Here's how the part is built. I have some questions about the finished solid (model axes, mm). A direction names the side the tool comes from. Give positions to 0.01 mm unless a question says otherwise; leave off trailing zeros. Loops run counter-clockwise (first coordinate to the right, second up) from the corner with the lowest first, then second, coordinate; pieces in that order, holes last. Notation, with made-up numbers: (-18, 30.5) - (29, 30.5) arc R14 ccw to (29, 36.5) - close; hole circle Ø8 at (75, 41). An arc over 180 degrees is marked (long way). Put each result on its own line as item: value. Start each with the question number.
from build123d import *


# Not quite as in the source:
# - a fillet or chamfer that OpenCascade refuses, or shapes differently, is made with other operations: its cross-section is extruded or revolved along the edge and cut away or added


with BuildPart() as f1:
    # F0 (on Front) → F1 (revolve)
    with BuildSketch(Plane.XZ):
        Polygon((-30, 7), (-30, 0), (0, 0), (0, 50), (-11.6, 50), (-11.6, 52.4), (-16, 52.4), (-16, 50), (-14.085106383, 48.085106383), (-16, 5), (-25, 5), (-25, 7), align=None)
    revolve(axis=Axis((0, 0, 15.8572417056), (0, 0, 1)))

    # F2: fillet of radius 3 on 5 edges, made by hand

    # F2_s1 → F2_t2 (revolve)
    with BuildSketch(Plane.XZ):
        with BuildLine():
            ThreePointArc((-22.1715728753, 5), (-23.9036236828, 5.5505102572), (-25, 7))
            Line((-25, 7), (-25, 5))
            Line((-25, 5), (-22.1715728753, 5))
        make_face()
    revolve(axis=Axis((0, 0, 5), (0, 0, 1)))

    # F2_s3 → F2_t4 (revolve)
    with BuildSketch(Plane.XZ):
        with BuildLine():
            ThreePointArc((-14.1437787706, 46.764977662), (-14.3443716648, 47.9844003118), (-15.0194998464, 49.0194998464))
            Line((-15.0194998464, 49.0194998464), (-14.085106383, 48.085106383))
            Line((-14.085106383, 48.085106383), (-14.1437787706, 46.764977662))
        make_face()
    revolve(axis=Axis((0, 0, 48.085106383), (0, 0, 1)))

    # F2_s5 → F2_t6 (revolve)
    with BuildSketch(Plane.XZ):
        with BuildLine():
            ThreePointArc((-8.6606123087, 50), (-10.5579789048, 50.6762099923), (-11.6, 52.4))
            Line((-11.6, 52.4), (-11.6, 50))
            Line((-11.6, 50), (-8.6606123087, 50))
        make_face()
    revolve(axis=Axis((0, 0, 50), (0, 0, 1)))

    # F2_s7 → F2_t8 (revolve, cut)
    with BuildSketch(Plane.XZ):
        with BuildLine():
            ThreePointArc((-27, 7), (-29.1213203436, 6.1213203436), (-30, 4))
            Line((-30, 4), (-30, 7))
            Line((-30, 7), (-27, 7))
        make_face()
    revolve(axis=Axis((0, 0, 7), (0, 0, 1)), mode=Mode.SUBTRACT)

    # F2_s9 → F2_t10 (revolve, cut)
    with BuildSketch(Plane.XZ):
        with BuildLine():
            ThreePointArc((-16, 50), (-14.9579789048, 51.7237900077), (-13.0606123087, 52.4))
            Line((-13.0606123087, 52.4), (-16, 52.4))
            Line((-16, 52.4), (-16, 50))
        make_face()
    revolve(axis=Axis((0, 0, 52.4), (0, 0, 1)), mode=Mode.SUBTRACT)


solid = f1.part
1) I'm going to push flat-ended pins straight in: P1, Ø12, axis at x = 0, y = -21.5, coming from the +Z side; P2, Ø6, axis at x = 1.5, z = 21, coming from the +Y side; P3, Ø8, axis at x = 5, z = 38.5, coming from the -Y side. Where does each tip first touch, or does it pass through?
2) Thinking about a two-plate mould opening in Y: for faces 1 (the flat face through (0, 0, 50)), 2 (the flat face through (0, -12, 52.4)), 3 (the cylindrical face through (29.97, -1.32, 1.97)), which applies, pulls with the +Y half, pulls with the -Y half, needs draft (parallel to the pull), parting line crosses it, or undercut?
3) Suppose I cut it at B-B on x = 0. Please give me the cut outline in (y, z).
4) Suppose I cut it at A-A on z = 32. Please give me the cut outline in (x, y).
5) Suppose I cut it at D-D on z = 13.5. Please give me the cut outline in (x, y), plus the area to 3 significant figures.
6) Which directions (+Z, -Z, +X, -X, +Y, -Y) give clear straight access to the entire face, cutting with the end or side of a thin tool? Please do faces 4 (the flat face through (0, 0, 0)), 5 (the conical face through (3.27, 14.726, 25.59)), 6 (the flat face through (6, 15, 5)).
7) I need wall thicknesses on line 1 (Y direction, x = -9, z = 6); line 2 (Z direction, x = -17, y = -7); line 3 (Z direction, x = -13, y = -24). Which ranges of each line are inside material? Lowest first, please.
Ans:
1. P1: stops at z = 51.15
1. P2: stops at y = 15.41
1. P3: stops at y = -14.52
2. face 1: undercut
2. face 2: needs draft
2. face 3: parting line crosses it
3. outline: (-30, 0) - (30, 0) - (30, 4) arc R3 ccw to (27, 7) - (25, 7) arc R3 cw to (22.17, 5) - (16, 5) - (14.14, 46.76) arc R3 cw to (15.02, 49.02) - (16, 50) arc R3 ccw to (13.06, 52.4) - (11.6, 52.4) arc R3 cw to (8.66, 50) - (-8.66, 50) arc R3 cw to (-11.6, 52.4) - (-13.06, 52.4) arc R3 ccw to (-16, 50) - (-15.02, 49.02) arc R3 cw to (-14.14, 46.76) - (-16, 5) - (-22.17, 5) arc R3 cw to (-25, 7) - (-27, 7) arc R3 ccw to (-30, 4) - close
4. outline: circle Ø29.6 at (0, 0)
5. outline: circle Ø31.24 at (0, 0)
5. area: 767 mm²
6. face 4: -Z, +X, -X, +Y, -Y
6. face 5: none
6. face 6: +Z
7. line 1: y = -27.82 to -22.69, -13.17 to 13.17, 22.69 to 27.82
7. line 2: z = 0 to 5
7. line 3: z = 0 to 6.99
